```python
from build123d import *

# Parameters (mm, degrees)
EXTRUDE_1_DEPTH     = 5
SKETCH_1_5_W        = 7
SKETCH_1_5_H        = 2.5
SKETCH_1_5_W_2      = 2.5
SKETCH_1_5_H_2      = 7
EXTRUDE_2_DEPTH     = 25
SKETCH_15_R         = 2.3
CUT_EXTRUDE_1_DEPTH = 20


with BuildPart() as part:
    # 草图1 → 凸台-拉伸1 (new body)
    with BuildSketch(Plane(origin=(0, 0, 0), x_dir=(1, 0, 0), z_dir=(0, 1, 0))):
        Polygon((-110, 150), (-150, 110), (-150, -110), (-110, -150), (110, -150), (150, -110), (150, 110), (110, 150), align=None)
    extrude(amount=EXTRUDE_1_DEPTH)

    # 草图1<5> → 凸台-拉伸2 (add)
    with BuildSketch(Plane(origin=(0, 0, 0), x_dir=(1, 0, 0), z_dir=(0, 1, 0))):
        with Locations((-36.5, -139.25)):
            Rectangle(SKETCH_1_5_W, SKETCH_1_5_H)
        with Locations((36.5, -139.25)):
            Rectangle(SKETCH_1_5_W, SKETCH_1_5_H)
        with Locations((139.25, 36.5)):
            Rectangle(SKETCH_1_5_W_2, SKETCH_1_5_H_2)
        with Locations((83.5, 139.25)):
            Rectangle(SKETCH_1_5_W, SKETCH_1_5_H)
        with Locations((-83.5, -139.25)):
            Rectangle(SKETCH_1_5_W, SKETCH_1_5_H)
        with Locations((83.5, -139.25)):
            Rectangle(SKETCH_1_5_W, SKETCH_1_5_H)
        with Locations((139.25, -83.5)):
            Rectangle(SKETCH_1_5_W_2, SKETCH_1_5_H_2)
        with Locations((139.25, -36.5)):
            Rectangle(SKETCH_1_5_W_2, SKETCH_1_5_H_2)
        with Locations((139.25, 83.5)):
            Rectangle(SKETCH_1_5_W_2, SKETCH_1_5_H_2)
        with Locations((36.5, 139.25)):
            Rectangle(SKETCH_1_5_W, SKETCH_1_5_H)
        with Locations((-139.25, 83.5)):
            Rectangle(SKETCH_1_5_W_2, SKETCH_1_5_H_2)
        with Locations((-139.25, 36.5)):
            Rectangle(SKETCH_1_5_W_2, SKETCH_1_5_H_2)
        with Locations((-83.5, 139.25)):
            Rectangle(SKETCH_1_5_W, SKETCH_1_5_H)
        with Locations((-36.5, 139.25)):
            Rectangle(SKETCH_1_5_W, SKETCH_1_5_H)
        with Locations((-139.25, -36.5)):
            Rectangle(SKETCH_1_5_W_2, SKETCH_1_5_H_2)
        with Locations((-139.25, -83.5)):
            Rectangle(SKETCH_1_5_W_2, SKETCH_1_5_H_2)
    extrude(amount=EXTRUDE_2_DEPTH)

    # 草图15 → 切除-拉伸1 (cut)
    with BuildSketch(Plane(origin=(0, 0, -140.5), x_dir=(-1, 0, 0), z_dir=(0, 0, -1))):
        with Locations((-83.5, 20)):
            Circle(SKETCH_15_R)
        with Locations((-83.5, 10)):
            Circle(SKETCH_15_R)
        with Locations((-36.5, 20)):
            Circle(SKETCH_15_R)
        with Locations((-36.5, 10)):
            Circle(SKETCH_15_R)
        with Locations((36.5, 10)):
            Circle(SKETCH_15_R)
        with Locations((36.5, 20)):
            Circle(SKETCH_15_R)
        with Locations((83.5, 20)):
            Circle(SKETCH_15_R)
        with Locations((83.5, 10)):
            Circle(SKETCH_15_R)
    extrude(amount=-CUT_EXTRUDE_1_DEPTH, mode=Mode.SUBTRACT)


solid = part.part
```
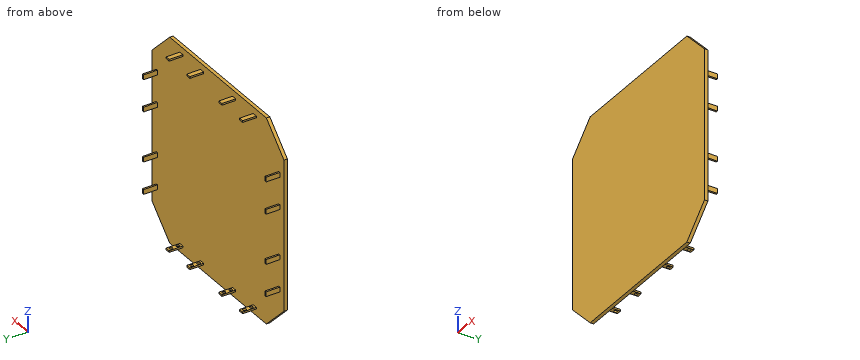
Can you work these out from the model? Positions are in its coordinate system, mm. Coordinates: 2 decimals unless noted, no trailing zeros. Loops run counter-clockwise (first coordinate to the right, second up) from the corner with the lowest first, then second, coordinate; pieces in that order, holes last. Notation, with made-up numbers: M 1.25,-27.75 L 12.25,-27.75 A21 ccw 12.25,5.25 Z; hole C 20.25,27.5 d6. An arc over 180 degrees is marked long. Put each result on its own line as item: value. Start each with the question number.
(1) Imagine slicing it at B-B on z = -55. List the corners of the cut face in (x, y) for me.
(2) I need wall thicknesses on probe 1 along Y at (x, z) = (36, -139) (3 decimals); probe 2 along Y at (x, z) = (-43, -117). Which ranges of each line are inside material? Lowest first, please.
(3) Imagine slicing it at A-A on x = 102.5. List the corners of the cut face in (y, z) for me.
(4) Will these pins go through, and if not, where does the flat tip stop? pin 1 Ø7.5 at (x, y) = (36.5, 16.5) entering from +Z; pin 2 Ø8 at (x, y) = (-108, 10.5) entering from +Z; pin 3 Ø0.8 at (x, y) = (-140, 16) entering from +Z; pin 4 Ø2 at (x, z) = (22.5, -21) entering from +Y.
Worked answers:
1. outline: M -150,0 L 150,0 L 150,5 L -150,5 Z
2. probe 1: y = 0 to 7.755, 12.245 to 17.755, 22.245 to 25
2. probe 2: y = 0 to 5
3. outline: M 0,-150 L 5,-150 L 5,150 L 0,150 Z
4. pin 1: stops at z = 140.5
4. pin 2: passes through
4. pin 3: stops at z = 87
4. pin 4: stops at y = 5
